For this review, take the finished solid that the model builds, in its own axes (mm). Face numbers are marked on the shaded views. A direction names the side the tool comes from. Give positions to 0.01 mm unless a question says otherwise; leave off trailing zeros. Loops run counter-clockwise (first coordinate to the right, second up) from the corner with the lowest first, then second, coordinate; pieces in that order, holes last. Notation, with made-up numbers: (36, -24.5) -> (82, -24.5) arc R11 ccw to (82, -16.5) -> close; hole circle Ø9 at (31, -37). An arc over 180 degrees is marked (long way). One line per question, with ' | ' between items. Start each with the question number.
(1) Draft analysis for pull direction X (two halves, no side actions). For the marked faces 1, 2 and 3, state which applies: +X half, -X half, draft (parallel to the pull), parting line (faces both ways), or undercut.
(2) Tool access review of the marked faces 4, 5, 6, 7 and 8: name each direction out of +Z, -Z, +X, -X, +Y, -Y from which nothing blocks a thin tool from reaching the whole face with its end or side.
(3) Insertion check: P1, Ø2, axis at x = 11.5, y = -13, coming from the -Z side; P2, Ø3, axis at x = -20, y = 21.5, coming from the -Z side; P3, Ø8, axis at x = 3, y = 3.5, coming from the +Z side. Each pin has a flat end and moves straight along its axis. Give the tip position at first contact, or say it passes through.
(4) Consider section B-B (x = 6). Write out the cut boundary in (y, z), and give its area (3 significant figures).
(5) Consider section A-A (z = 9). Write out the cut boundary in (x, y).
(6) Wall thickness on probe 1 along Y at (x, z) = (19.85, 1.45); probe 2 along Y at (x, z) = (-19, 34); probe 3 along Y at (x, z) = (27, 31): over which ranges is each line inside the solid? List them lowest first.
from build123d import *

# Parameters (mm, degrees)
SKETCH_W        = 65.5
SKETCH_H        = 65.5
PAD_DEPTH       = 37
SKETCH001_W     = 25.5
SKETCH001_H     = 14
POCKET_DEPTH    = 65.501
SKETCH002_W     = 25.5
SKETCH002_H     = 14
POCKET001_DEPTH = 65.501
CHAMFER_1_SIZE2 = 18
CHAMFER_1_SIZE  = 20
CHAMFER_2_SIZE2 = 18
CHAMFER_2_SIZE  = 20
CHAMFER_3_SIZE2 = 18
CHAMFER_3_SIZE  = 20
CHAMFER_4_SIZE2 = 18
CHAMFER_4_SIZE  = 20
SKETCH003_R     = 5
POCKET002_DEPTH = 2.5
SKETCH004_R     = 3.5
SKETCH004_R_2   = 2.45
PAD001_DEPTH    = 2
SKETCH005_R     = 2
POCKET003_DEPTH = 10
CHAMFER001_SIZE = 0.25
POCKET004_DEPTH = 3
SKETCH007_R     = 2.05
POCKET005_DEPTH = 12
POCKET006_DEPTH = 1.575
SKETCH009_R     = 2
POCKET007_DEPTH = 5


with BuildPart() as part:
    # Sketch → Pad (new body)
    with BuildSketch(Plane.XY):
        Rectangle(SKETCH_W, SKETCH_H)
    extrude(amount=PAD_DEPTH)

    # Sketch001 (on Face3 of Pad) → Pocket (cut, through all)
    with BuildSketch(Plane.XZ.offset(32.75)):
        with Locations((0, 30)):
            Rectangle(SKETCH001_W, SKETCH001_H)
    extrude(amount=-POCKET_DEPTH, mode=Mode.SUBTRACT)

    # Sketch002 (on Face9 of Pocket) → Pocket001 (cut, through all)
    with BuildSketch(Plane(origin=(-32.75, 0, 0), x_dir=(0, -1, 0), z_dir=(-1, 0, 0))):
        with Locations((0, 30)):
            Rectangle(SKETCH002_W, SKETCH002_H)
    extrude(amount=-POCKET001_DEPTH, mode=Mode.SUBTRACT)

    # Chamfer 1
    chamfer_1_edges = [part.edges().sort_by_distance(p)[0] for p in [
        (0, 32.75, 23),
    ]]
    chamfer_1_side = part.faces().sort_by_distance((0, 32.75, 16.513308))[0]
    chamfer(chamfer_1_edges, length=CHAMFER_1_SIZE, length2=CHAMFER_1_SIZE2, reference=chamfer_1_side)

    # Chamfer 2
    chamfer_2_edges = [part.edges().sort_by_distance(p)[0] for p in [
        (0, -32.75, 23),
    ]]
    chamfer_2_side = part.faces().sort_by_distance((0, -32.75, 16.513308))[0]
    chamfer(chamfer_2_edges, length=CHAMFER_2_SIZE, length2=CHAMFER_2_SIZE2, reference=chamfer_2_side)

    # Chamfer 3
    chamfer_3_edges = [part.edges().sort_by_distance(p)[0] for p in [
        (-32.75, 0, 23),
    ]]
    chamfer_3_side = part.faces().sort_by_distance((-32.75, 0, 16.513308))[0]
    chamfer(chamfer_3_edges, length=CHAMFER_3_SIZE, length2=CHAMFER_3_SIZE2, reference=chamfer_3_side)

    # Chamfer 4
    chamfer_4_edges = [part.edges().sort_by_distance(p)[0] for p in [
        (32.75, 0, 23),
    ]]
    chamfer_4_side = part.faces().sort_by_distance((32.75, 0, 16.513308))[0]
    chamfer(chamfer_4_edges, length=CHAMFER_4_SIZE, length2=CHAMFER_4_SIZE2, reference=chamfer_4_side)

    # Sketch003 (on Face7 of Chamfer) → Pocket002 (cut)
    with BuildSketch(Plane(origin=(0, 0, 0), x_dir=(1, 0, 0), z_dir=(0, 0, -1))):
        with Locations((-19.85, 20)):
            Circle(SKETCH003_R)
        with Locations((19.85, 20)):
            Circle(SKETCH003_R)
        with Locations((-19.85, -20)):
            Circle(SKETCH003_R)
        with Locations((19.85, -20)):
            Circle(SKETCH003_R)
    extrude(amount=-POCKET002_DEPTH, mode=Mode.SUBTRACT)

    # Sketch004 (on Face7 of Pocket002) → Pad001 (join)
    with BuildSketch(Plane(origin=(0, 0, 0), x_dir=(1, 0, 0), z_dir=(0, 0, -1))):
        with Locations((-19.85, 0)):
            Circle(SKETCH004_R)
        with Locations((19.85, 0)):
            Circle(SKETCH004_R_2)
    extrude(amount=PAD001_DEPTH)

    # Sketch005 (on Face34 of Pad001) → Pocket003 (cut)
    with BuildSketch(Plane(origin=(0, 0, -2), x_dir=(1, 0, 0), z_dir=(0, 0, -1))):
        with Locations((-19.85, 0)):
            Circle(SKETCH005_R)
        with Locations((19.85, 0)):
            Circle(SKETCH005_R)
    extrude(amount=-POCKET003_DEPTH, mode=Mode.SUBTRACT)

    # Chamfer001
    chamfer001_edges = [part.edges().sort_by_distance(p)[0] for p in [
        (-23.35, 0, -2),
        (17.4, 0, -2),
    ]]
    chamfer(chamfer001_edges, length=CHAMFER001_SIZE)

    # Sketch006 (on Face36 of Chamfer001) → Pocket004 (cut)
    with BuildSketch(Plane(origin=(0, 0, 8), x_dir=(1, 0, 0), z_dir=(0, 0, -1))):
        Polygon((-19.85, -4), (-16.385898, -2), (-16.385898, 2), (-19.85, 4), (-23.314102, 2), (-23.314102, -2), align=None)
        Polygon((19.85, -4), (23.314102, -2), (23.314102, 2), (19.85, 4), (16.385898, 2), (16.385898, -2), align=None)
    extrude(amount=POCKET004_DEPTH, mode=Mode.SUBTRACT)

    # Sketch007 (on Face22 of Pocket004) → Pocket005 (cut)
    with BuildSketch(Plane.XY.offset(37)):
        with Locations((-19.85, 20)):
            Circle(SKETCH007_R)
        with Locations((19.85, 20)):
            Circle(SKETCH007_R)
        with Locations((-19.85, -20)):
            Circle(SKETCH007_R)
        with Locations((19.85, -20)):
            Circle(SKETCH007_R)
    extrude(amount=-POCKET005_DEPTH, mode=Mode.SUBTRACT)

    # Sketch008 (on DatumPlane) → Pocket006 (cut, symmetric)
    with BuildSketch(Plane.XY.offset(32)):
        Polygon((-19.85, 16), (-16.385898, 18), (-16.385898, 22), (-19.85, 24), (-23.314102, 22), (-23.314102, 18), align=None)
        Polygon((-19.85, -24), (-16.385898, -22), (-16.385898, -18), (-19.85, -16), (-23.314102, -18), (-23.314102, -22), align=None)
        Polygon((19.85, 16), (23.314102, 18), (23.314102, 22), (19.85, 24), (16.385898, 22), (16.385898, 18), align=None)
        Polygon((19.85, -24), (23.314102, -22), (23.314102, -18), (19.85, -16), (16.385898, -18), (16.385898, -22), align=None)
    extrude(amount=POCKET006_DEPTH, both=True, mode=Mode.SUBTRACT)

    # Sketch009 (on Face104 of Pocket006) → Pocket007 (cut)
    with BuildSketch(Plane(origin=(0, 0, 8), x_dir=(1, 0, 0), z_dir=(0, 0, -1))):
        with Locations((-19.85, 0)):
            Circle(SKETCH009_R)
        with Locations((19.85, 0)):
            Circle(SKETCH009_R)
    extrude(amount=-POCKET007_DEPTH, mode=Mode.SUBTRACT)


solid = part.part
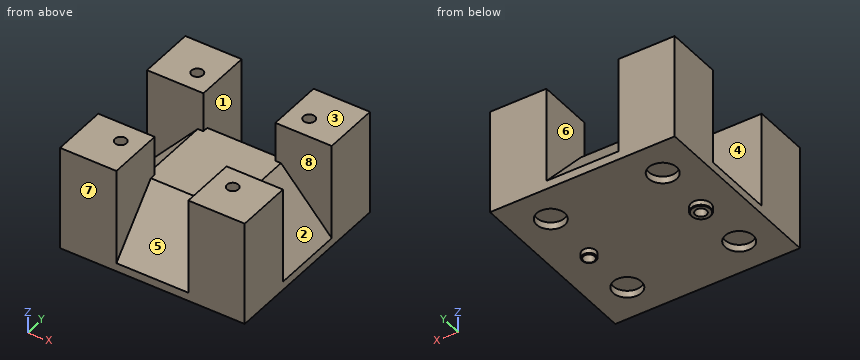
A:
1) face 1: undercut | face 2: +X half | face 3: draft
2) face 4: +Z, -X | face 5: +Z, -Y | face 6: +Z, +Y | face 7: +Z, -Z, +X, -X, -Y | face 8: +Z, +X
3) P1: stops at z = 0 | P2: stops at z = 2.5 | P3: stops at z = 23
4) outline: (-32.75, 0) -> (32.75, 0) -> (32.75, 3) -> (14.75, 23) -> (-14.75, 23) -> (-32.75, 3) -> close | area: 1,150 mm^2
5) outline: (-32.75, -32.75) -> (-12.75, -32.75) -> (-12.75, -27.35) -> (12.75, -27.35) -> (12.75, -32.75) -> (32.75, -32.75) -> (32.75, -12.75) -> (27.35, -12.75) -> (27.35, 12.75) -> (32.75, 12.75) -> (32.75, 32.75) -> (12.75, 32.75) -> (12.75, 27.35) -> (-12.75, 27.35) -> (-12.75, 32.75) -> (-32.75, 32.75) -> (-32.75, 12.75) -> (-27.35, 12.75) -> (-27.35, -12.75) -> (-32.75, -12.75) -> close; hole circle Ø4 at (-19.85, 0); hole circle Ø4 at (19.85, 0)
6) probe 1: y = -32.75 to -25, -15 to -2, 2 to 15, 25 to 32.75 | probe 2: y = -32.75 to -21.87, -18.13 to -12.75, 12.75 to 18.13, 21.87 to 32.75 | probe 3: y = -32.75 to -12.75, 12.75 to 32.75
